```python
from build123d import *

# Parameters (mm, degrees)
F1_DEPTH = 63.5
F2_DEPTH = 63.5
F3_DEPTH = 63.5


with BuildPart() as f1:
    # F0 (on Front) → F1 (new body, symmetric)
    with BuildSketch(Plane.XZ):
        Polygon((-41.275, 9.525), (-41.275, -9.525), (41.275, -9.525), (41.275, 9.525), (22.225, 9.525), align=None)
    extrude(amount=F1_DEPTH, both=True)

    # F0 (on Front) → F2 (join, symmetric)
    with BuildSketch(Plane.XZ):
        Polygon((-41.275, 9.525), (-41.275, -9.525), (41.275, -9.525), (41.275, 9.525), (22.225, 9.525), align=None)
        with BuildLine():
            add(Edge.make_bspline(
                [(-41.275, 9.525), (-35.113391, 45.455925), (13.393071, 65.25448), (57.15, 61.9252)],
                knots=[0, 0, 0, 0, 111.504536, 111.504536, 111.504536, 111.504536], degree=3))
            Line((-41.275, 9.525), (22.225, 9.525))
            Line((22.225, 9.525), (22.225, 27.0002))
            ThreePointArc((22.225, 27.0002), (32.454296, 51.695904), (57.15, 61.9252))
        make_face()
        with BuildLine():
            Line((22.225, 9.525), (41.275, 9.525))
            Line((41.275, 9.525), (41.275, 27.0002))
            ThreePointArc((41.275, 27.0002), (45.92468, 38.22552), (57.15, 42.8752))
            Line((57.15, 42.8752), (63.200993, 42.8752))
            Line((63.200993, 42.8752), (63.200993, 61.9252))
            Line((63.200993, 61.9252), (57.15, 61.9252))
            ThreePointArc((57.15, 61.9252), (32.454296, 51.695904), (22.225, 27.0002))
            Line((22.225, 27.0002), (22.225, 9.525))
        make_face()
        Polygon((63.200993, 66.675), (63.200993, 61.9252), (63.200993, 42.8752), (87.960352, 42.8752), (88.600993, 66.675), align=None)
        Polygon((87.960352, 42.8752), (63.200993, 42.8752), (63.200993, 34.925), (114.000993, 34.925), (114.000993, 66.675), (88.600993, 66.675), align=None)
    extrude(amount=F2_DEPTH, both=True)

    # F1_face (on face) → F3 (join, symmetric)
    with BuildSketch(Plane(origin=(-41.275, 0, 0), x_dir=(0, -1, 0), z_dir=(-1, 0, 0))):
        Polygon((-63.5, 9.525), (-63.5, -9.525), (63.5, -9.525), (63.5, 9.525), (0, 9.525), align=None)
    extrude(amount=F3_DEPTH, both=True)


solid = f1.part
```
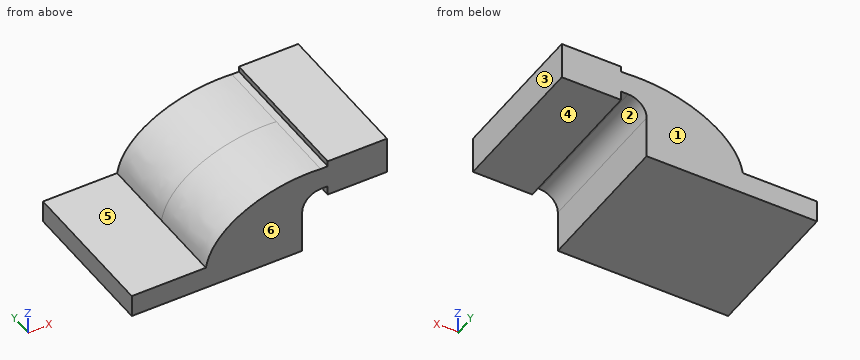
Verification items for the finished model (mm, model axes). Face numbers are marked on the shaded views. A direction names the side the tool comes from. Give positions to 0.01 mm unless a question says otherwise; leave off trailing zeros. Order: outer loops, then holes, each group sorted by start corner. A loop starts at its lowest first (then second) coordinate and runs counter-clockwise, first axis right, second up. Notation, with made-up numbers: (-26, -40) -> (12, -40) arc R12 ccw to (12, -24) -> close; hole circle Ø5 at (38.5, 40). An arc over 180 degrees is marked (long way). Use a Markdown table: item, result.
1) Depth check by flat-ended pin: pin 1 Ø4 at (y, z) = (8, 11.5) entering from +X (3 decimals); pin 2 Ø5 at (x, y) = (61.5, -18) entering from -Z (3 decimals); pin 3 Ø6.5 at (x, y) = (59.5, 24.5) entering from +Z. Enter the tip coordinate at first touch or a pass-through.
Results:
| item | result |
|---|---|
| pin 1 | x = 41.275 |
| pin 2 | z = 34.925 |
| pin 3 | z = 61.99 |
2) Tool access check on the marked faces 4, 5 and 6. Record the directions out of +Z, -Z, +X, -X, +Y, -Y that give a thin tool (end or side, any length) a straight path to the whole face; none if there is none.
Results:
| item | result |
|---|---|
| face 4 | -Z, +X, +Y, -Y |
| face 5 | +Z, -X, +Y, -Y |
| face 6 | +Z, -Z, +X, -X, -Y |
3) Section check B-B, the plane x = -74. Record the boundary of the cut face in (y, z) (3 decimals), then the cut area to 3 significant figures.
Results:
| item | result |
|---|---|
| outline | (-63.5, -9.525) -> (63.5, -9.525) -> (63.5, 9.525) -> (-63.5, 9.525) -> close |
| area | 2,420 mm² |
4) Section check A-A, the plane z = -1. Record the boundary of the cut face in (x, y) (3 decimals), then the cut area to 3 significant figures.
Results:
| item | result |
|---|---|
| outline | (-104.775, -63.5) -> (41.275, -63.5) -> (41.275, 63.5) -> (-104.775, 63.5) -> close |
| area | 18,500 mm² |
5) Mould release check, pull along X, two halves, no side actions. Record for the marked faces 1, 2 and 3: pulls with the +X half, pulls with the -X half, needs draft (parallel to the pull), parting line crosses it, or undercut.
Results:
| item | result |
|---|---|
| face 1 | needs draft |
| face 2 | undercut |
| face 3 | pulls with the +X half |
6) Material ranges on probe 1 along Z at (x, y) = (92, 12) (3 decimals); probe 2 along X at (y, z) = (-40, -3) (3 decimals); probe 3 along Z at (x, y) = (56.5, -7.5), recorded low to high.
Results:
| item | result |
|---|---|
| probe 1 | 34.925 to 66.675 |
| probe 2 | -104.775 to 41.275 |
| probe 3 | 42.86 to 61.97 |
